Input: part model. Units: mm. Frame: model coordinates. Face numbers are marked on the shaded views. A direction names the side the tool comes from. Coordinates: 2 decimals unless noted, no trailing zeros. Order: outer loops, then holes, each group sorted by start corner. A loop starts at its lowest first (then second) coordinate and runs counter-clockwise, first axis right, second up. Notation, with made-up numbers: M -24,-21.75 L 33,-21.75 A15 cw 33,-0.75 Z; hole C -7,64 d9. An arc over 180 degrees is marked long. Answer in a Markdown table with one row per item.
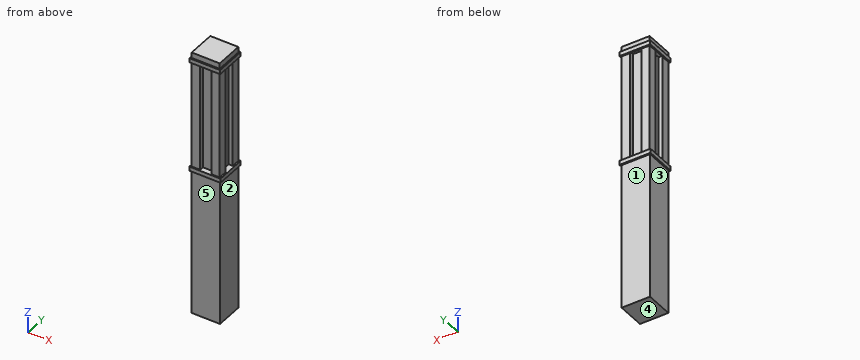
from build123d import *

# Parameters (mm, degrees)
F0_W      = 128.778
F0_H      = 125.476
F1_DEPTH  = 673.1
F2_W      = 88.9
F2_H      = 88.9
F3_DEPTH  = 508
F4_W      = 141.477994
F4_H      = 138.175994
F4_W_2    = 88.9
F4_H_2    = 88.9
F5_DEPTH  = 12.7
F6_W      = 141.477994
F6_H      = 138.175994
F6_W_2    = 128.778
F6_H_2    = 125.476
F7_DEPTH  = 6.35
F8_W      = 38.1
F8_H      = 38.1
F9_DEPTH  = 495.3
F10_W     = 139.7
F10_H     = 139.7
F10_W_2   = 127
F10_H_2   = 127
F11_DEPTH = 6.35
F12_W     = 139.7
F12_H     = 139.7
F13_DEPTH = 12.7
F14_W     = 127
F14_H     = 127
F15_DEPTH = 25.4


with BuildPart() as f1:
    # F0 (on Top) → F1 (new body)
    with BuildSketch(Plane.XY):
        Rectangle(F0_W, F0_H)
    extrude(amount=F1_DEPTH)

    # F2 (on face) → F3 (join)
    with BuildSketch(Plane.XY.offset(673.1)):
        Rectangle(F2_W, F2_H)
    extrude(amount=F3_DEPTH)

    # F4 (on face) → F5 (join)
    with BuildSketch(Plane.XY.offset(673.1)):
        Rectangle(F4_W, F4_H)
        Rectangle(F4_W_2, F4_H_2, mode=Mode.SUBTRACT)
    extrude(amount=F5_DEPTH)

    # F6 (on face) → F7 (join)
    with BuildSketch(Plane(origin=(0, 0, 673.1), x_dir=(1, 0, 0), z_dir=(0, 0, -1))):
        Rectangle(F6_W, F6_H)
        Rectangle(F6_W_2, F6_H_2, mode=Mode.SUBTRACT)
    extrude(amount=F7_DEPTH)

    # F8 (on face) → F9 (join)
    with BuildSketch(Plane.XY.offset(685.8)):
        with Locations((44.45, 44.45)):
            Rectangle(F8_W, F8_H)
        with Locations((44.45, -44.45)):
            Rectangle(F8_W, F8_H)
        with Locations((-44.45, -44.45)):
            Rectangle(F8_W, F8_H)
        with Locations((-44.45, 44.45)):
            Rectangle(F8_W, F8_H)
    extrude(amount=F9_DEPTH)

    # F10 (on face) → F11 (join)
    with BuildSketch(Plane.XY.offset(1181.1)):
        Rectangle(F10_W, F10_H)
        Rectangle(F10_W_2, F10_H_2, mode=Mode.SUBTRACT)
    extrude(amount=-F11_DEPTH)

    # F12 (on face) → F13 (join)
    with BuildSketch(Plane.XY.offset(1181.1)):
        Rectangle(F12_W, F12_H)
    extrude(amount=F13_DEPTH)

    # F14 (on face) → F15 (join)
    with BuildSketch(Plane.XY.offset(1193.8)):
        Rectangle(F14_W, F14_H)
    extrude(amount=F15_DEPTH)


solid = f1.part
1) Cut plane C-C, the plane z = 934. Output: boundary loops of the cut face in (x, y).
Resolved:
| item | result |
|---|---|
| outline | M -63.5,-63.5 L -25.4,-63.5 L -25.4,-44.45 L 25.4,-44.45 L 25.4,-63.5 L 63.5,-63.5 L 63.5,-25.4 L 44.45,-25.4 L 44.45,25.4 L 63.5,25.4 L 63.5,63.5 L 25.4,63.5 L 25.4,44.45 L -25.4,44.45 L -25.4,63.5 L -63.5,63.5 L -63.5,25.4 L -44.45,25.4 L -44.45,-25.4 L -63.5,-25.4 Z |
2) Contact query for flat-ended pins moving along their axis: pin 1 (5 mm diameter, centred on x = 36, z = 319, fed in from -Y); pin 2 (11.5 mm diameter, centred on x = 50, z = 980, fed in from -Y); pin 3 (12.5 mm diameter, centred on y = 26.5, z = 1208, fed in from -X). Output: stop coordinate, or through.
Resolved:
| item | result |
|---|---|
| pin 1 | stops at y = -62.74 |
| pin 2 | stops at y = -63.5 |
| pin 3 | stops at x = -63.5 |
3) Cut plane A-A, the plane y = 9.5. Output: boundary loops of the cut face in (x, z).
Resolved:
| item | result |
|---|---|
| outline | M -70.74,666.75 L -64.39,666.75 L -64.39,0 L 64.39,0 L 64.39,666.75 L 70.74,666.75 L 70.74,685.8 L 44.45,685.8 L 44.45,1181.1 L 63.5,1181.1 L 63.5,1174.75 L 69.85,1174.75 L 69.85,1193.8 L 63.5,1193.8 L 63.5,1219.2 L -63.5,1219.2 L -63.5,1193.8 L -69.85,1193.8 L -69.85,1174.75 L -63.5,1174.75 L -63.5,1181.1 L -44.45,1181.1 L -44.45,685.8 L -70.74,685.8 Z |
4) Cut plane D-D, the plane z = 610. Output: boundary loops of the cut face in (x, y), and give its area (3 significant figures).
Resolved:
| item | result |
|---|---|
| outline | M -64.39,-62.74 L 64.39,-62.74 L 64.39,62.74 L -64.39,62.74 Z |
| area | 16,200 mm2 |
5) Cut plane B-B, the plane x = -3.5. Output: boundary loops of the cut face in (y, z).
Resolved:
| item | result |
|---|---|
| outline | M -69.85,1174.75 L -63.5,1174.75 L -63.5,1181.1 L -44.45,1181.1 L -44.45,685.8 L -69.09,685.8 L -69.09,666.75 L -62.74,666.75 L -62.74,0 L 62.74,0 L 62.74,666.75 L 69.09,666.75 L 69.09,685.8 L 44.45,685.8 L 44.45,1181.1 L 63.5,1181.1 L 63.5,1174.75 L 69.85,1174.75 L 69.85,1193.8 L 63.5,1193.8 L 63.5,1219.2 L -63.5,1219.2 L -63.5,1193.8 L -69.85,1193.8 Z |
6) Material intervals for probe 1 along Y at (x, z) = (61, 729); probe 2 along Z at (x, y) = (15, -57.5); probe 3 along X at (y, z) = (4.5, 1078), sorted ascending.
Resolved:
| item | result |
|---|---|
| probe 1 | y = -63.5 to -25.4, 25.4 to 63.5 |
| probe 2 | z = 0 to 685.8, 1181.1 to 1219.2 |
| probe 3 | x = -44.45 to 44.45 |
7) Reachability of the marked faces 1, 2, 3, 4 and 5 from +Z, -Z, +X, -X, +Y, -Y: full face, straight path, thin tool, end or side. Return the list, or none.
Resolved:
| item | result |
|---|---|
| face 1 | -Z, +X, -X, +Y |
| face 2 | -Z, +X, +Y, -Y |
| face 3 | -Z, -X, +Y, -Y |
| face 4 | -Z, +X, -X, +Y, -Y |
| face 5 | -Z, +X, -X, -Y |
